Read the model definition and answer for the solid it produces. Units are mm, in the model's axes. Coordinates: 2 decimals unless noted, no trailing zeros. Write each loop counter-clockwise with the first axis right and the second up, starting at its lowest first coordinate (ties: lowest second). Pieces come first, ordered by that corner, then holes. Notation, with made-up numbers: (18, -13) -> (44, -13) arc R29 ccw to (44, 12) -> close; hole circle Ø6 at (82.5, -22.75). An arc over 180 degrees is marked (long way). Return JSON: item names as keys, results as strings.
from build123d import *

# Parameters (mm, degrees)
BOSS_EXTRUDE1_DEPTH = 1.5
FILLET5_R           = 2


with BuildPart() as part:
    # Sketch1 → Boss-Extrude1 (new, symmetric)
    with BuildSketch(Plane(origin=(0, 0, 0), x_dir=(1, 0, 0), z_dir=(0, 1, 0))):
        Polygon((-14.297771125, -12.5), (14.297771125, -12.5), (22.216878365, -12.5), (7.783121635, 12.5), (-7.783121635, 12.5), (-22.216878365, -12.5), align=None)
    extrude(amount=BOSS_EXTRUDE1_DEPTH, both=True)

    # Fillet5
    fillet5_edges = [part.edges().sort_by_distance(p)[0] for p in [
        (-22.216878365, 0, 12.5),
        (-7.783121635, 0, -12.5),
        (7.783121635, 0, -12.5),
        (22.216878365, 0, 12.5),
    ]]
    fillet(fillet5_edges, radius=FILLET5_R)


solid = part.part
1. Consider L1, parallel to X at y = -0.25, z = -3.5; L2, parallel to X at y = -1.3, z = -6.25; L3, parallel to Z at x = 9, y = -0.8. Determine where each line is inside the solid, lowest interval first.
Taken from the geometry:
{"L1": "x = -12.98 to 12.98", "L2": "x = -11.39 to 11.39", "L3": "z = -10.39 to 12.5"}
2. A flat-ended cylindrical pin translates along its axis: pin 1 Ø1 at (y, z) = (-1, 5.5) entering from -X. Find the tip coordinate at first contact, or state that the pin passes through.
Taken from the geometry:
{"pin 1": "stops at x = -18.46"}
3. The part is cut by section A-A (y = 0.9). Determine the outline of the cut face in (x, z).
Taken from the geometry:
{"outline": "(-20.48, 9.5) -> (-8.36, -11.5) arc R2 ccw to (-6.63, -12.5) -> (6.63, -12.5) arc R2 ccw to (8.36, -11.5) -> (20.48, 9.5) arc R2 ccw to (18.75, 12.5) -> (-18.75, 12.5) arc R2 ccw to start"}
4. The part is cut by section C-C (x = -11.5). Determine the outline of the cut face in (y, z), then the cut area to 3 significant figures.
Taken from the geometry:
{"outline": "(-1.5, -6.06) -> (1.5, -6.06) -> (1.5, 12.5) -> (-1.5, 12.5) -> close", "area": "55.7 mm2"}
5. The part is cut by section B-B (z = 0). Determine the outline of the cut face in (x, y).
Taken from the geometry:
{"outline": "(-15, -1.5) -> (15, -1.5) -> (15, 1.5) -> (-15, 1.5) -> close"}
